Drawing for the job (mm, zero at the part's lowest x, y, z). Round coordinates to 2 decimals unless told otherwise and drop trailing zeros. Loops run counter-clockwise (first coordinate to the right, second up) from the corner with the lowest first, then second, coordinate; pieces in that order, holes last. Notation, with made-up numbers: M 6,-19 L 28,-19 A27 ccw 28,7 Z; hole C -25,59.5 d1. An arc over 180 degrees is marked long. Put each result on its own line as item: value. Start each with the question number.
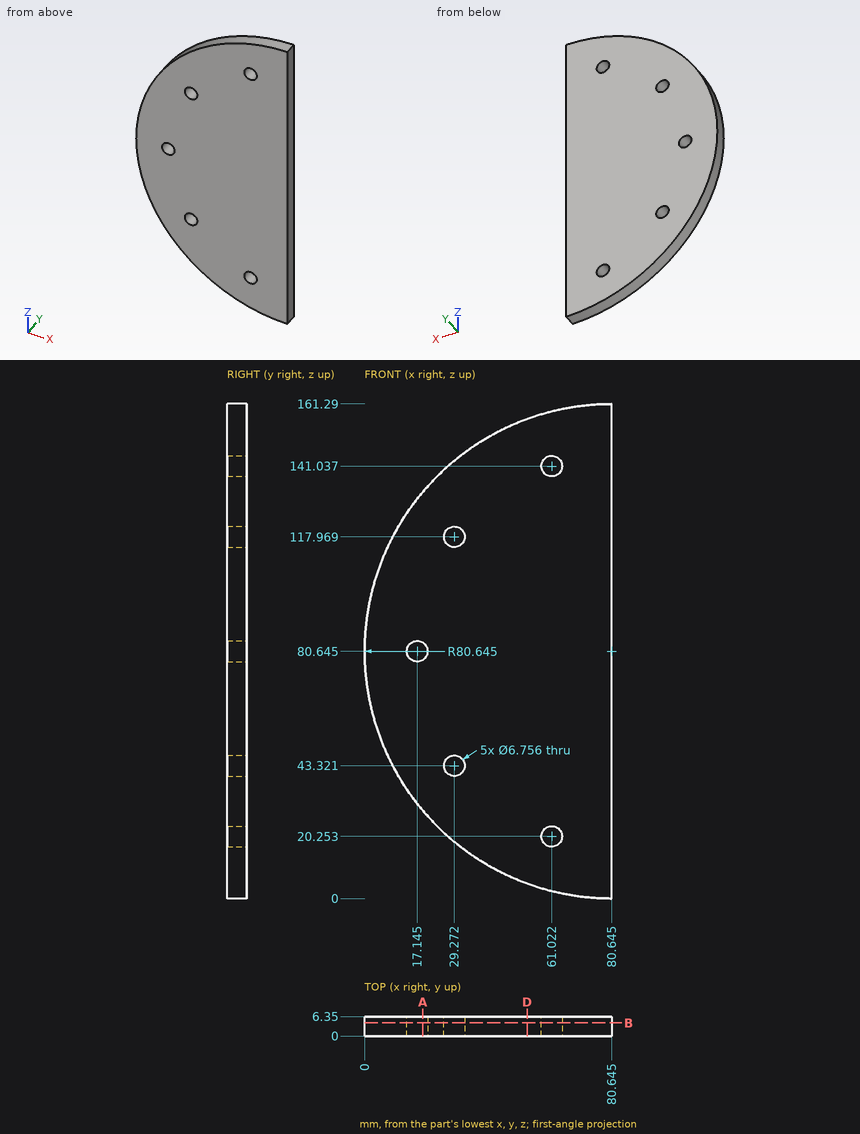
1. Cut at A-A, the plane x = 19. Give the cut face in (y, z).
2. Drop a flat-ended pin along its axis: pin 1 (1.5 mm diameter, centred on x = 67.5, y = 4, fed in from +Z). Give the stop position or say it passes through.
3. Cut at D-D, the plane x = 53. Give the cut face in (y, z), and give its area (3 significant figures).
4. Wall check: L1, parallel to X at y = 1, z = 72 (1 decimal); L2, parallel to Z at x = 13, y = 2.25; L3, parallel to Z at x = 9, y = 1.75 (1 decimal). Give the ranges that are in metal, low to high.
5. Cut at B-B, the plane y = 4.25. Give the number of separate pieces and of enclosed holes in the cut face, and give its area (3 significant figures).
Results list:
1. outline: M 0,28.65 L 6.35,28.65 L 6.35,77.82 L 0,77.82 Z; M 0,83.47 L 6.35,83.47 L 6.35,132.64 L 0,132.64 Z
2. pin 1: stops at z = 160.33
3. outline: M 0,4.89 L 6.35,4.89 L 6.35,156.4 L 0,156.4 Z
3. area: 962 mm^2
4. L1: x = 0.5 to 80.6
4. L2: z = 36.74 to 124.55
4. L3: z = 43.6 to 117.7
5. separate pieces: 1
5. enclosed holes: 5
5. area: 10,000 mm^2
